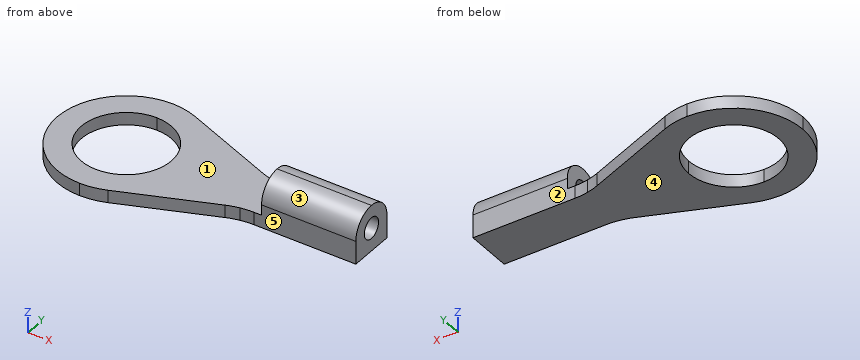
```python
from build123d import *

# Parameters (mm, degrees)
F0_W     = 4.5
F0_H     = 2.2
F1_DEPTH = 0.6
F2_W     = 4.5
F2_H     = 2.2
F3_DEPTH = 1.6
F4_R     = 1.09999
F5_R     = 0.5
F6_DEPTH = 25


# Not quite as in the source:
# - a fillet or chamfer is up to 0.001 mm smaller than in the source, because OpenCascade refuses the exact size


with BuildPart() as f1:
    # F0 (on Top) → F1 (new body)
    with BuildSketch(Plane.XY):
        with BuildLine():
            ThreePointArc((8.9159970588, 1.9694225865), (9.2040660975, 2.0680561106), (9.5, 2.1397182935))
            Line((9.5, 2.1397182935), (9.5, 4.4602817065))
            ThreePointArc((9.5, 4.4602817065), (9.2040660975, 4.5319438894), (8.9159970588, 4.6305774135))
            Line((8.9159970588, 4.6305774135), (4.5118766379, 6.3694225865))
            ThreePointArc((4.5118766379, 6.3694225865), (3.9168085053, 6.5418431899), (3.3, 6.6))
            Line((3.3, 6.6), (3.3, 5.45))
            ThreePointArc((3.3, 5.45), (4.8202795796, 4.8202795796), (5.45, 3.3))
            ThreePointArc((5.45, 3.3), (4.8202795796, 1.7797204204), (3.3, 1.15))
            Line((3.3, 1.15), (3.3, 0))
            ThreePointArc((3.3, 0), (3.9168085053, 0.0581568101), (4.5118766379, 0.2305774135))
            Line((4.5118766379, 0.2305774135), (8.9159970588, 1.9694225865))
        make_face()
        with Locations((12.75, 3.3)):
            Rectangle(F0_W, F0_H)
        with BuildLine():
            Line((10.1278736967, 2.2), (10.5, 2.2))
            Line((10.5, 2.2), (10.5, 4.4))
            Line((10.5, 4.4), (10.1278736967, 4.4))
            ThreePointArc((10.1278736967, 4.4), (9.8124932664, 4.4151049965), (9.5, 4.4602817065))
            Line((9.5, 4.4602817065), (9.5, 2.1397182935))
            ThreePointArc((9.5, 2.1397182935), (9.8124932664, 2.1848950035), (10.1278736967, 2.2))
        make_face()
        with BuildLine():
            ThreePointArc((0, 3.3), (0.9665476221, 0.9665476221), (3.3, 0))
            Line((3.3, 0), (3.3, 1.15))
            ThreePointArc((3.3, 1.15), (1.15, 3.3), (3.3, 5.45))
            Line((3.3, 5.45), (3.3, 6.6))
            ThreePointArc((3.3, 6.6), (0.9665476221, 5.6334523779), (0, 3.3))
        make_face()
    extrude(amount=F1_DEPTH)

    # F2 (on face) → F3 (join)
    with BuildSketch(Plane.XY.offset(0.6)):
        with Locations((12.75, 3.3)):
            Rectangle(F2_W, F2_H)
    extrude(amount=F3_DEPTH)

    # F4 (radius 1.1 in the source; OpenCascade refuses exactly that, so slightly less here)
    f4_edges = [f1.edges().sort_by_distance(p)[0] for p in [
        (12.75, 4.4, 2.2),
        (12.75, 2.2, 2.2),
    ]]
    fillet(f4_edges, radius=F4_R)

    # F5 (on face) → F6 (cut)
    with BuildSketch(Plane.YZ.offset(15)):
        with Locations((3.3, 1.1)):
            Circle(F5_R)
    extrude(amount=-F6_DEPTH, mode=Mode.SUBTRACT)


solid = f1.part
```
Can you work these out from the model? Positions are in its coordinate system, mm. Face numbers are marked on the shaded views. A direction names the side the tool comes from. Give positions to 0.01 mm unless a question says otherwise; leave off trailing zeros. Order: outer loops, then holes, each group sorted by start corner. A loop starts at its lowest first (then second) coordinate and runs counter-clockwise, first axis right, second up. Notation, with made-up numbers: (-15.5, 82.5) - (38.5, 82.5) arc R33 cw to (38.5, 121.5) - close; hole circle Ø6 at (-27, 89.25). An arc over 180 degrees is marked (long way). Use a Markdown table: item, result. Add a question column.
Q1. Please list where these lines run through material, in increasing order: line 1 along Y through (x, z) = (13.95, 1.1); line 2 along Z through (x, y) = (11.5, 3.3); line 3 along Z through (x, y) = (5.75, 4.5).
Q2. I'm going to push flat-ended pins straight in: pin 1 (0.9 mm diameter, centred on x = 12.5, z = 0.5, fed in from -Y); pin 2 (2 mm diameter, centred on x = 5, y = 2.5, fed in from +Z); pin 3 (1.3 mm diameter, centred on y = 3, z = 1.5, fed in from -X). Where does each tip first touch, or does it pass through?
Q3. If we mould it in two halves opening along Y, with no side actions, what happens to the marked faces 1, 2 and 3? For each: released by +Y, released by -Y, zero draft, split by the parting line, or undercut.
Q4. If we section it at C-C on x = 5: Write out the boundary of the cut face in (y, z), plus the area to 3 significant figures.
Q5. If we section it at A-A on y = 1.5: Write out the boundary of the cut face in (x, z), plus the area to 3 significant figures.
Q6. On a 3-axis mill with a long thin cutter (end or side, diameter ignored), from which of +Z, -Z, +X, -X, +Y, -Y can I reach the whole of each face in a straight line? I mean the marked faces 4 and 5. Say none if no direction works.
Q7. If we section it at D-D on y = 2.5: Write out the boundary of the cut face in (x, z).
Answers follow:
| question | item | result |
|---|---|---|
| 1 | line 1 | y = 2.2 to 2.8, 3.8 to 4.4 |
| 1 | line 2 | z = 0 to 0.6, 1.6 to 2.2 |
| 1 | line 3 | z = 0 to 0.6 |
| 2 | pin 1 | stops at y = 2.2 |
| 2 | pin 2 | stops at z = 0.6 |
| 2 | pin 3 | stops at x = 10.5 |
| 3 | face 1 | zero draft |
| 3 | face 2 | released by +Y |
| 3 | face 3 | released by -Y |
| 4 | outline | (0.42, 0) - (1.98, 0) - (1.98, 0.6) - (0.42, 0.6) - close; (4.62, 0) - (6.18, 0) - (6.18, 0.6) - (4.62, 0.6) - close |
| 4 | area | 1.87 mm^2 |
| 5 | outline | (0.53, 0) - (2.12, 0) - (2.12, 0.6) - (0.53, 0.6) - close; (4.48, 0) - (7.73, 0) - (7.73, 0.6) - (4.48, 0.6) - close |
| 5 | area | 2.90 mm^2 |
| 6 | face 4 | -Z, +X, -X, +Y, -Y |
| 6 | face 5 | +Z, -Z, +X, -Y |
| 7 | outline | (0.1, 0) - (1.3, 0) - (1.3, 0.6) - (0.1, 0.6) - close; (5.3, 0) - (15, 0) - (15, 1.85) - (10.5, 1.85) - (10.5, 0.6) - (5.3, 0.6) - close |
